Geometry: final body of the model. Coordinates: model frame, mm. Round coordinates to 2 decimals unless told otherwise and drop trailing zeros. Order: outer loops, then holes, each group sorted by start corner. A loop starts at its lowest first (then second) coordinate and runs counter-clockwise, first axis right, second up. Notation, with made-up numbers: (61.5, -20.5) -> (91.5, -20.5) arc R21 cw to (91.5, -11.5) -> close; hole circle Ø9 at (-11.5, 58.5). An arc over 180 degrees is marked (long way). Put each result on its own line as item: value.
```python
from build123d import *

# Parameters (mm, degrees)
F0_W     = 600
F0_H     = 500
F0_R     = 42.5
F1_DEPTH = 5


with BuildPart() as f1:
    # F0 (on Front) → F1 (new body)
    with BuildSketch(Plane.XZ):
        with Locations((-240.587708, 259.897342)):
            Rectangle(F0_W, F0_H)
        with BuildLine():
            ThreePointArc((-418.087708, 234.897342), (-481.732182, 208.013955), (-456.632586, 272.382782))
            ThreePointArc((-456.632586, 272.382782), (-429.443234, 261.780728), (-418.087708, 234.897342))
        make_face(mode=Mode.SUBTRACT)
        with Locations((-240.587708, 234.897342)):
            Circle(F0_R, mode=Mode.SUBTRACT)
        with BuildLine():
            ThreePointArc((-526.886874, 450.694124), (-522.637445, 452.22814), (-518.12026, 452.15139))
            ThreePointArc((-518.12026, 452.15139), (-516.144254, 451.580908), (-514.288543, 450.694124))
            ThreePointArc((-514.288543, 450.694124), (-509.748207, 446.12271), (-508.087708, 439.897342))
            ThreePointArc((-508.087708, 439.897342), (-510.868779, 432.036526), (-517.974496, 427.673548))
            ThreePointArc((-517.974496, 427.673548), (-532.244607, 435.384393), (-526.886874, 450.694124))
        make_face(mode=Mode.SUBTRACT)
        with BuildLine():
            ThreePointArc((-270.587708, 439.897342), (-280.235755, 422.784859), (-299.871415, 422.18258))
            ThreePointArc((-299.871415, 422.18258), (-300.939661, 457.009825), (-270.587708, 439.897342))
        make_face(mode=Mode.SUBTRACT)
        with BuildLine():
            ThreePointArc((-371.770186, 476.479024), (-351.197542, 477.555903), (-340.587708, 459.897342))
            ThreePointArc((-340.587708, 459.897342), (-369.977874, 442.238781), (-371.770186, 476.479024))
        make_face(mode=Mode.SUBTRACT)
        with BuildLine():
            ThreePointArc((-170.587708, 439.897342), (-173.475225, 429.545389), (-181.304001, 422.18258))
            ThreePointArc((-181.304001, 422.18258), (-207.700191, 450.249295), (-170.587708, 439.897342))
        make_face(mode=Mode.SUBTRACT)
        with BuildLine():
            ThreePointArc((-100.587708, 459.897342), (-138.246269, 450.507175), (-109.405231, 476.479024))
            ThreePointArc((-109.405231, 476.479024), (-102.929147, 469.287508), (-100.587708, 459.897342))
        make_face(mode=Mode.SUBTRACT)
        with BuildLine():
            ThreePointArc((51.912292, 439.897342), (47.273108, 430.178413), (36.79908, 427.673548))
            ThreePointArc((36.79908, 427.673548), (27.069507, 437.921069), (33.113126, 450.694124))
            ThreePointArc((33.113126, 450.694124), (34.968838, 451.580908), (36.944844, 452.15139))
            ThreePointArc((36.944844, 452.15139), (41.462029, 452.22814), (45.711457, 450.694124))
            ThreePointArc((45.711457, 450.694124), (50.251793, 446.12271), (51.912292, 439.897342))
        make_face(mode=Mode.SUBTRACT)
    extrude(amount=F1_DEPTH)


solid = f1.part
```
1. Draft query along X for faces 1 (the face through (-217.74, -2.465, 270.734)), 2 (the face through (-245, 0, 319)). Return one class per face: +X half, -X half, draft (parallel to the pull), parting line (faces both ways), or undercut.
Ans:
face 1: undercut
face 2: draft
2. Cut plane C-C on x = -430. Return loops of the section in (y, z), and give its area (3 significant figures).
Ans:
outline: (-5, 9.9) -> (0, 9.9) -> (0, 207.48) -> (-5, 207.48) -> close; (-5, 262.31) -> (0, 262.31) -> (0, 509.9) -> (-5, 509.9) -> close
area: 2,230 mm²
3. Cut plane B-B on z = 466.5. Return loops of the section in (x, y), and give its area (3 significant figures).
Ans:
outline: (-540.59, -5) -> (-379.47, -5) -> (-379.47, 0) -> (-540.59, 0) -> close; (-341.71, -5) -> (-139.47, -5) -> (-139.47, 0) -> (-341.71, 0) -> close; (-101.71, -5) -> (59.41, -5) -> (59.41, 0) -> (-101.71, 0) -> close
area: 2,620 mm²
4. Material intervals for probe 1 along Z at (x, y) = (-193, -2.55); probe 2 along X at (y, z) = (-4.8, 454); probe 3 along Z at (x, y) = (-239.5, -0.8), sorted ascending.
Ans:
probe 1: 9.9 to 420.04, 459.75 to 509.9
probe 2: -540.59 to -379.7, -341.48 to -304.77, -276.41 to -204.77, -176.41 to -139.7, -101.48 to 59.41
probe 3: 9.9 to 192.41, 277.38 to 509.9
5. Cut plane A-A on y = -3.15. State how many separate pieces and enclosed holes the cut face has, and give its area (3 significant figures).
Ans:
separate pieces: 1
enclosed holes: 8
area: 284,000 mm²
6. Cut plane D-D on z = 266. Return loops of the section in (x, y).
Ans:
outline: (-540.59, -5) -> (-476.54, -5) -> (-476.54, 0) -> (-540.59, 0) -> close; (-434.64, -5) -> (-269.55, -5) -> (-269.55, 0) -> (-434.64, 0) -> close; (-211.62, -5) -> (59.41, -5) -> (59.41, 0) -> (-211.62, 0) -> close
